Source: three-view drawing plus pictorial views. Frame: mm from the lowest corner of the part. Give positions to 0.01 mm unless a question says otherwise; leave off trailing zeros. Loops run counter-clockwise (first coordinate to the right, second up) from the corner with the lowest first, then second, coordinate; pieces in that order, holes last.
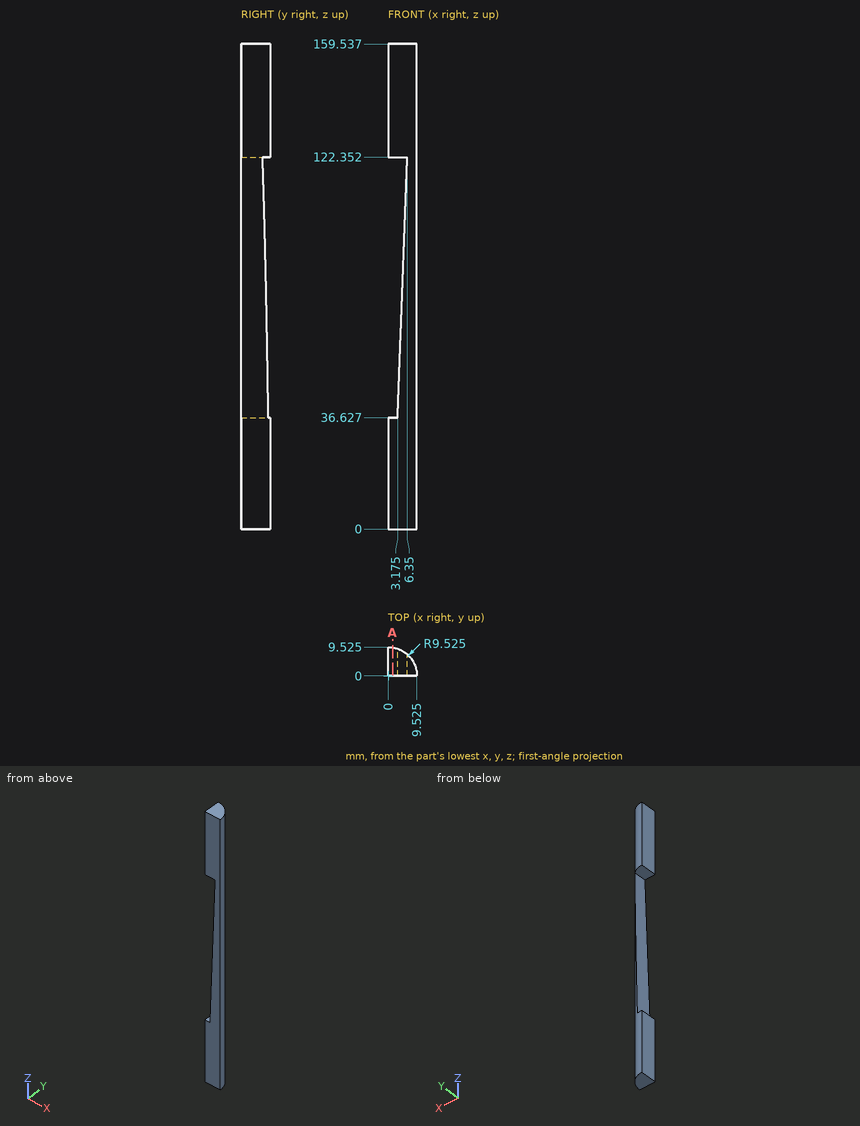
1) Ray query, probe 1 along Z at (x, y) = (1.25, 0.75); probe 2 along Y at (x, z) = (1.25, 149.5); probe 3 along X at (y, z) = (6.5, 21). Return the intervals inside material, ascending.
Checks:
probe 1: z = 0 to 36.63, 122.35 to 159.54
probe 2: y = 0 to 9.44
probe 3: x = 0 to 6.96
2) Cut plane A-A (x = 1.5). Return loops of the section in (y, z), and give its area (3 significant figures).
Checks:
outline: (0, 0) - (9.41, 0) - (9.41, 36.63) - (0, 36.63) - close; (0, 122.35) - (9.41, 122.35) - (9.41, 159.54) - (0, 159.54) - close
area: 694 mm2
3) Contact query for flat-ended pins moving along their axis: P1, Ø5, axis at y = 4.5, z = 114.5, coming from the +X side; P2, Ø3, axis at y = 8, z = 117.5, coming from the +X side; P3, Ø1, axis at x = 7, z = 33.5, coming from the +Y side. Output: stop coordinate, or through.
Checks:
P1: stops at x = 9.31
P2: stops at x = 6.96
P3: stops at y = 6.96
